Autodesk Inventor part; units mm, degrees
ref_plane "YZ Plane" through (0, 0, 0) normal (1, 0, 0) x (0, 1, 0)
ref_plane "XZ Plane" through (0, 0, 0) normal (0, 1, 0) x (-1, 0, 0)
ref_plane "XY Plane" through (0, 0, 0) normal (0, 0, 1) x (1, 0, 0)
sketch "Sketch1" plane through (0, 0, 0) normal (0, 1, 0) x (-1, 0, 0)
  line L0 (7.1515, 37.8857) -> (-18.2485, 37.8857)
  line L1 (-18.2485, 37.8857) -> (-18.2485, -12.9143)
  line L2 (-18.2485, -12.9143) -> (7.1515, -12.9143)
  line L3 (7.1515, -12.9143) -> (7.1515, 37.8857)
  point P0 (0, 0)
  dimension "d0" = 25.4
  dimension "d1" = 50.8
extrude "Extrusion1" add sketch "Sketch1" along normal blind 406.4
chamfer "Chamfer1" distance 43.18 angle 45 2 edges at (5.5485, 406.4, 37.8857) (5.5485, 0, 37.8857)
sketch "Sketch2" plane through (-7.1515, 43.18, 37.8857) normal (0, 0, 1) x (1, 0, 0)
  circle A0 centre (12.7, 350.52) radius 3.175
  line L0 (25.4, 363.22) -> (0, 363.22)
  circle A1 centre (12.7, -30.48) radius 3.175
  line L1 (0, -43.18) -> (25.4, -43.18)
  point P0 (7.1515, -43.18)
  dimension "d7" = 6.35
  dimension "d8" = 12.7
  dimension "d9" = 6.35
  dimension "d10" = 12.7
hole "Hole1" at (5.5485, 393.7, 37.8857) at (5.5485, 12.7, 37.8857) direction (0, 0, -1) diameter 6.35 end through all
properties part number "slanted_alum_bar"
Model file for the job. Use its own axes, mm. Give positions to 0.01 mm unless a question says otherwise; leave off trailing zeros. Write each loop counter-clockwise with the first axis right and the second up, starting at its lowest first coordinate (ties: lowest second). Pieces come first, ordered by that corner, then holes. Notation, with made-up numbers: M 45,69 L 50,69 A19 ccw 50,88 Z; hole C -15,15 d6. An arc over 180 degrees is marked long. One line per item, written item: value. Start each with the question number.
Q1. Saw through at A-A, the plane x = 14.25. Write the cut outline in (y, z), plus the area to 3 significant figures.
Q2. Probe probe 1 along X at (y, z) = (12.7, -1.75); probe 2 along Y at (x, z) = (-5, 24); probe 3 along Y at (x, z) = (-1, 23). List the from-to ranges inside material, lowest first. Write a range as [from, to].
Q3. Drop flat-ended pins along their axis: pin 1 Ø10 at (x, y) = (5.55, 393.7) entering from +Z; pin 2 Ø12 at (x, z) = (1, 8) entering from +Y; pin 3 Ø5.5 at (x, y) = (5.55, 12.7) entering from -Z; pin 4 Ø5 at (x, z) = (6, 1) entering from +Y. Give the stop position or say it passes through.
Q4. Two-plate mould, pull along Y, no slides. Class faces 1 (the flat face through (6, 200, -12.914)), 2 (the cylindrical face through (5.41, 15.87, -3.93)), 3 (the flat face through (5.726, 385.112, 15.993)), 4 (the cylindrical face through (4.595, 390.672, -1.33)): +Y half, -Y half, draft (parallel to the pull), parting line (faces both ways), or undercut.
Q5. Saw through at C-C, the plane z = 33. Write the cut outline in (x, y).
Q6. Saw through at B-B, the plane z = -1. State how many separate pieces and enclosed holes the cut face has, plus the area to 3 significant figures.
Output values:
1. outline: M 0,-12.91 L 406.4,-12.91 L 406.4,-5.29 L 363.22,37.89 L 43.18,37.89 L 0,-5.29 Z
1. area: 18,800 mm²
2. probe 1: x = [-7.15, 2.37], [8.72, 18.25]
2. probe 2: y = [29.29, 377.11]
2. probe 3: y = [28.29, 378.11]
3. pin 1: stops at z = 12.41
3. pin 2: stops at y = 399.11
3. pin 3: passes through
3. pin 4: stops at y = 402.61
4. face 1: draft
4. face 2: undercut
4. face 3: +Y half
4. face 4: undercut
5. outline: M -7.15,38.29 L 18.25,38.29 L 18.25,368.11 L -7.15,368.11 Z
6. separate pieces: 1
6. enclosed holes: 2
6. area: 10,000 mm²
